Design review of the part built by this model. Coordinates are the model's own, in mm. A direction names the side the tool comes from. Give positions to 0.01 mm unless a question says otherwise; leave off trailing zeros. Write each loop counter-clockwise with the first axis right and the second up, starting at its lowest first coordinate (ties: lowest second). Pieces come first, ordered by that corner, then holes. Notation, with made-up numbers: M 65.5,64.5 L 78.5,64.5 A24 ccw 78.5,94.5 Z; hole C 32,12.5 d5. An arc over 180 degrees is marked long. Answer in a Markdown table with one row per item.
Autodesk Inventor part; units mm, degrees
ref_plane "YZ Plane" through (0, 0, 0) normal (1, 0, 0) x (0, 1, 0)
ref_plane "XZ Plane" through (0, 0, 0) normal (0, 1, 0) x (-1, 0, 0)
ref_plane "XY Plane" through (0, 0, 0) normal (0, 0, 1) x (1, 0, 0)
sketch "Sketch1" plane through (0, 0, 0) normal (0, 1, 0) x (-1, 0, 0)
  line L0 (-38.1, 25.4) -> (38.1, 25.4)
  line L1 (38.1, 25.4) -> (38.1, -25.4)
  line L2 (38.1, -25.4) -> (-38.1, -25.4)
  line L3 (-38.1, -25.4) -> (-38.1, 25.4)
  line L4 (-38.1, 25.4) -> (38.1, -25.4) construction
  line L5 (38.1, 25.4) -> (-38.1, -25.4) construction
  point P0 (0, 0)
  dimension "d0" = 76.2
  dimension "d1" = 50.8
extrude "Extrusion1" add sketch "Sketch1" along normal blind 12.7
sketch "Sketch2" plane through (0, 12.7, 0) normal (0, 1, 0) x (1, 0, 0)
  line L0 (-38.1, 25.4) -> (-38.1, -25.4)
  line L1 (-38.1, 6.35) -> (-25.4, 6.35)
  line L2 (-25.4, 6.35) -> (-25.4, -6.35)
  line L3 (-25.4, -6.35) -> (-38.1, -6.35)
  line L4 (-38.1, -6.35) -> (-38.1, 6.35)
  point P0 (0, 0)
  dimension "d4" = 12.7
  dimension "d5" = 12.7
  dimension "d6" = 6.35
extrude "Extrusion2" add sketch "Sketch2" along normal blind 63.5
sketch "Sketch4" plane through (-38.1, 12.7, 6.35) normal (0, 0, 1) x (1, 0, 0)
  line L0 (0, 0) -> (0, 63.5)
  line L1 (0, 50.8) -> (-12.7, 50.8)
  line L2 (-12.7, 50.8) -> (-12.7, 76.2)
  line L3 (-12.7, 76.2) -> (0, 76.2)
  line L4 (0, 76.2) -> (0, 50.8)
  line L5 (0, 63.5) -> (12.7, 63.5)
  line L6 (-12.7, 50.8) -> (0, 31.75)
  circle A0 centre (-6.35, 69.85) radius 3.175
  point P0 (38.1, -12.7)
  dimension "d13" = 12.7
  dimension "d14" = 25.4
  dimension "d15" = 12.7
  dimension "d22" = 6.35
  dimension "d23" = 6.35
  dimension "d24" = 6.35
extrude "Extrusion4" add sketch "Sketch4" against normal blind 12.7
sketch "Sketch5" plane through (-50.8, 88.9, 6.35) normal (0, 1, 0) x (1, 0, 0)
  line L0 (0, 0) -> (0, 12.7)
  line L1 (12.7, 12.7) -> (12.7, 0)
  line L2 (0, 9.525) -> (12.7, 9.525)
  line L3 (12.7, 9.525) -> (12.7, 3.175)
  line L4 (12.7, 3.175) -> (0, 3.175)
  line L5 (0, 3.175) -> (0, 9.525)
  line L6 (12.7, 0) -> (0, 0)
  point P0 (50.8, 6.35)
  point P1 (0, 3.175)
  dimension "d18" = 6.35
  dimension "d19" = 3.175
extrude "Extrusion5" cut sketch "Sketch5" against normal blind 12.7 contours L0 L2 L1 L4
sketch "Sketch6" plane through (38.1, 0, 25.4) normal (1, 0, 0) x (0, 0, -1)
  line L0 (15.875, 8.89) -> (34.925, 8.89)
  line L1 (34.925, 8.89) -> (34.925, 5.08)
  line L2 (34.925, 5.08) -> (15.875, 5.08)
  line L3 (15.875, 5.08) -> (15.875, 8.89)
  line L4 (50.8, 0) -> (50.8, 12.7)
  line L5 (0, 12.7) -> (50.8, 12.7)
  line L6 (21.59, 8.89) -> (29.21, 8.89)
  line L7 (29.21, 8.89) -> (29.21, 12.7)
  line L8 (29.21, 12.7) -> (21.59, 12.7)
  line L9 (21.59, 12.7) -> (21.59, 8.89)
  point P0 (25.4, 0)
  point P1 (29.21, 12.7)
  dimension "d25" = 19.05
  dimension "d26" = 3.81
  dimension "d27" = 15.875
  dimension "d28" = 3.81
  dimension "d29" = 7.62
  dimension "d30" = 3.81
  dimension "d31" = 5.715
extrude "Extrusion6" cut sketch "Sketch6" against normal blind 22.86
fillet "Fillet1" radius 7.62 2 edges at (-38.1, 88.9, 4.7625) (-38.1, 88.9, -4.7625)
properties part number "Press_Base"
1) For faces 5 (the face through (-47, 80, 3.175)), 6 (the face through (-1, 6, -25.4)), 7 (the face through (-35, 50, -6.35)), 8 (the face through (27, 7, -9.525)), 9 (the face through (27, 11, -3.81)), list the 3-axis set-ups (+Z, -Z, +X, -X, +Y, -Y) from which the entire face can be reached by the end or side of a thin tool; tool diameter is ignored.
Geometry says:
| item | result |
|---|---|
| face 5 | +X, -X, +Y |
| face 6 | -Z, +X, -X, +Y, -Y |
| face 7 | -Z, +X, -X, +Y |
| face 8 | +X |
| face 9 | +X, +Y |
2) To check wall thickness, follow probe 1 along Y at (x, z) = (-13.5, -18); probe 2 along X at (y, z) = (11, -0.5); probe 3 along X at (y, z) = (82, 4). State the ranges of each line that lie inside material, in increasing order. Write a range as [from, to].
Geometry says:
| item | result |
|---|---|
| probe 1 | [0, 12.7] |
| probe 2 | [-38.1, 15.24] |
| probe 3 | [-50.8, -47.58], [-41.32, -38.13] |
3) Add section C-C (y = 82.55). Write out the cut boundary in (x, z) (3 decimals), and give its area (3 significant figures).
Geometry says:
| item | result |
|---|---|
| outline | M -50.8,-6.35 L -47.625,-6.35 L -47.625,-3.175 L -50.8,-3.175 Z; M -50.8,3.175 L -47.625,3.175 L -47.625,6.35 L -50.8,6.35 Z; M -41.275,-6.35 L -38.207,-6.35 L -38.207,-3.175 L -41.275,-3.175 Z; M -41.275,3.175 L -38.207,3.175 L -38.207,6.35 L -41.275,6.35 Z |
| area | 39.6 mm^2 |
4) Insertion check: P1, Ø14, axis at x = -41.5, y = 80, coming from the +Z side; P2, Ø6.5, axis at y = 56, z = 3, coming from the +X side; P3, Ø9.5, axis at x = 26, z = -3.5, coming from the +Y side. Each pin has a flat end and moves straight along its axis. Give the tip position at first contact, or say it passes through.
Geometry says:
| item | result |
|---|---|
| P1 | z = 6.35 |
| P2 | x = -25.4 |
| P3 | y = 12.7 |
5) Add section A-A (x = -33). Write out the cut boundary in (y, z), and give its area (3 significant figures).
Geometry says:
| item | result |
|---|---|
| outline | M 0,-25.4 L 12.7,-25.4 L 12.7,-6.35 L 76.2,-6.35 L 76.2,6.35 L 12.7,6.35 L 12.7,25.4 L 0,25.4 Z |
| area | 1,450 mm^2 |
6) Add section D-D (x = -44.45). Write out the cut boundary in (y, z) (3 decimals), and give its area (3 significant figures).
Geometry says:
| item | result |
|---|---|
| outline | M 53.975,-6.35 L 79.375,-6.35 L 79.375,-3.175 L 76.2,-3.175 L 76.2,3.175 L 79.375,3.175 L 79.375,6.35 L 53.975,6.35 Z; M 85.725,-6.35 L 88.793,-6.35 L 88.793,-3.175 L 85.725,-3.175 Z; M 85.725,3.175 L 88.793,3.175 L 88.793,6.35 L 85.725,6.35 Z |
| area | 322 mm^2 |
7) The part is to be moulded in two halves that separate along X. For faces 1 (the face through (27, 8.89, -7)), 2 (the face through (-42.985, 79.733, -4.74)), 3 (the face through (-38.1, 17, 0)), 4 (the face through (-40.391, 86.727, 4.74)), say which applies: released by +X, released by -X, zero draft, split by the parting line, or undercut.
Geometry says:
| item | result |
|---|---|
| face 1 | zero draft |
| face 2 | undercut |
| face 3 | released by -X |
| face 4 | released by +X |
8) Add section B-B (z = -7.5). Write out the cut boundary in (x, y).
Geometry says:
| item | result |
|---|---|
| outline | M -38.1,0 L 38.1,0 L 38.1,5.08 L 15.24,5.08 L 15.24,8.89 L 38.1,8.89 L 38.1,12.7 L -38.1,12.7 Z |
